```python
from build123d import *

# Parameters (mm, degrees)
BOSS_EXTRUDE1_DEPTH = 1.75
SKETCH2_R           = 0.675
CUT_EXTRUDE4_DEPTH  = 15
SKETCH7_R           = 0.675
CUT_EXTRUDE8_DEPTH  = 15
SKETCH8_R           = 0.675
CUT_EXTRUDE9_DEPTH  = 15
SKETCH9_R           = 0.675
CUT_EXTRUDE10_DEPTH = 15
SKETCH10_R          = 0.675
CUT_EXTRUDE11_DEPTH = 15


with BuildPart() as part:
    # Sketch1 → Boss-Extrude1 (new body, symmetric)
    with BuildSketch(Plane(origin=(0, 0, 0), x_dir=(1, 0, 0), z_dir=(0, 1, 0))):
        Polygon((1.75, -2.408668361), (1.75, -17.408668361), (-1.75, -17.408668361), (-1.75, -2.408668361), (-16.015847744, -7.043923276), (-17.097407225, -3.715225469), (-2.83155948, 0.920029446), (-11.648338265, 13.055284362), (-8.816778784, 15.112532745), (0, 2.977277829), (8.816778784, 15.112532745), (11.648338265, 13.055284362), (2.83155948, 0.920029446), (17.097407225, -3.715225469), (16.015847744, -7.043923276), align=None)
    extrude(amount=BOSS_EXTRUDE1_DEPTH, both=True)

    # Sketch2 → Cut-Extrude4 (cut)
    with BuildSketch(Plane.XY.offset(17.408668361)):
        Circle(SKETCH2_R)
    extrude(amount=-CUT_EXTRUDE4_DEPTH, mode=Mode.SUBTRACT)

    # Sketch7 → Cut-Extrude8 (cut)
    with BuildSketch(Plane(origin=(16.556627485, 0, 5.379574373), x_dir=(0.309016994, 0, -0.951056516), z_dir=(0.951056516, 0, 0.309016994))):
        Circle(SKETCH7_R)
    extrude(amount=-CUT_EXTRUDE8_DEPTH, mode=Mode.SUBTRACT)

    # Sketch8 → Cut-Extrude9 (cut)
    with BuildSketch(Plane(origin=(10.232558525, 0, -14.083908553), x_dir=(-0.809016994, 0, -0.587785252), z_dir=(0.587785252, 0, -0.809016994))):
        Circle(SKETCH8_R)
    extrude(amount=-CUT_EXTRUDE9_DEPTH, mode=Mode.SUBTRACT)

    # Sketch9 → Cut-Extrude10 (cut)
    with BuildSketch(Plane(origin=(-10.232558525, 0, -14.083908553), x_dir=(-0.809016994, 0, 0.587785252), z_dir=(-0.587785252, 0, -0.809016994))):
        Circle(SKETCH9_R)
    extrude(amount=-CUT_EXTRUDE10_DEPTH, mode=Mode.SUBTRACT)

    # Sketch10 → Cut-Extrude11 (cut)
    with BuildSketch(Plane(origin=(-16.556627485, 0, 5.379574373), x_dir=(0.309016994, 0, 0.951056516), z_dir=(-0.951056516, 0, 0.309016994))):
        Circle(SKETCH10_R)
    extrude(amount=-CUT_EXTRUDE11_DEPTH, mode=Mode.SUBTRACT)


solid = part.part
```
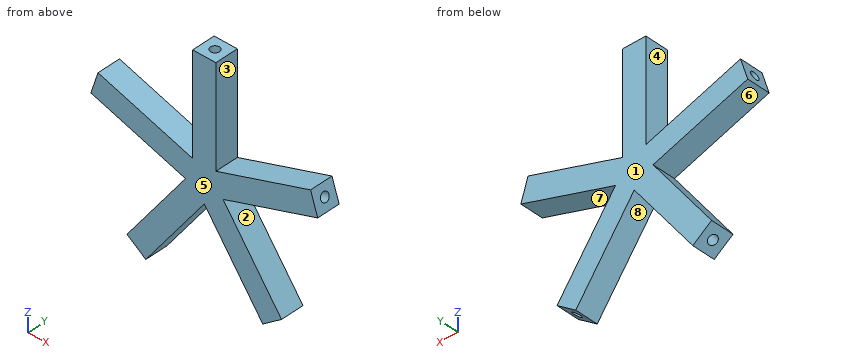
The listing builds one solid part. Answer for the finished solid, in the listing's coordinates (mm). Face numbers are marked on the shaded views. A direction names the side the tool comes from. Coordinates: 2 decimals unless noted, no trailing zeros. Loops run counter-clockwise (first coordinate to the right, second up) from the corner with the lowest first, then second, coordinate; pieces in that order, holes last. Notation, with made-up numbers: (57.5, 72.5) -> (109.5, 72.5) arc R34 ccw to (109.5, 105.5) -> close; hole circle Ø6 at (82, -12). An arc over 180 degrees is marked (long way). Return JSON: item names as keys, results as strings. Group by question number.
(1) A cutting plane is placed at C-C on z = -7.5. Count the separate pieces of the cut face and the enclosed holes in it, and give its area (3 significant figures).
(2) Find the intervals of material crossed by probe 1 along Y at (x, z) = (0, 14) (3 decimals); probe 2 along Z at (x, y) = (-11, -0.15); probe 3 along Z at (x, y) = (-10.5, 0.05), in increasing order. Write a range as from..to.
(3) Determine the mould class of the marked faces 1, 2 and 3 for opening direction X: released by +X, released by -X, zero draft, split by the parting line, or undercut.
(4) Given pin 1 Ø1.8 at (x, y) = (0, 0) entering from -Z; pin 2 Ø0.7 at (x, y) = (0, 0) entering from +Z, each flat-ended and moving along its own axis, determine where each tip first touches the part or whether it passes through.
(5) A cutting plane is placed at B-B on y = 1.1. Write down the section's boundary in (x, z).
(6) Which of the six approach directions +Z, -Z, +X, -X, +Y, -Y give full straight-line access (tool end or side, diameter ignored) to the marked faces 4, 5, 6, 7 and 8?
(7) A cutting plane is placed at A-A on z = 9. Write down the section's boundary in (x, y) (3 decimals), and give its area (3 significant figures).
The answers:
{
 "1": {"separate pieces": "2", "enclosed holes": "2", "area": "26.7 mm^2"},
 "2": {"probe 1": "y = -1.75..-0.675, 0.675..1.75", "probe 2": "z = -13.53..-12.16, 1.73..2.88, 4.27..5.41", "probe 3": "z = -13.31..-11.47, 1.57..2.7, 4.12..5.25"},
 "3": {"face 1": "zero draft", "face 2": "released by +X", "face 3": "undercut"},
 "4": {"pin 1": "stops at z = -4.22", "pin 2": "stops at z = 2.41"},
 "5": {"outline": "(-17.1, 3.72) -> (-2.83, -0.92) -> (-11.65, -13.06) -> (-8.82, -15.11) -> (0, -2.98) -> (8.82, -15.11) -> (11.65, -13.06) -> (2.83, -0.92) -> (17.1, 3.72) -> (16.02, 7.04) -> (1.75, 2.41) -> (1.75, 17.41) -> (-1.75, 17.41) -> (-1.75, 2.41) -> (-16.02, 7.04) -> close"},
 "6": {"face 4": "+Z, +Y, -Y", "face 5": "+Z, -Z, +X, -X, -Y", "face 6": "-X, +Y, -Y", "face 7": "+X, +Y, -Y", "face 8": "-Z, +Y, -Y"},
 "7": {"outline": "(-1.75, -1.75) -> (1.75, -1.75) -> (1.75, 1.75) -> (-1.75, 1.75) -> close; hole circle Ø1.35 at (0, 0)", "area": "10.8 mm^2"}
}
